from build123d import *

# Parameters (mm, degrees)
SKETCH001_R = 2.2
PAD_DEPTH   = 3
FILLET_R    = 5


with BuildPart() as part:
    # Sketch001 → Pad (new body)
    with BuildSketch(Plane.XY):
        Polygon((3.9, -6), (-3.9, -6), (-3.9, -2), (-5.9, -2), (-5.9, 13), (5.9, 13), (5.9, -2), (3.9, -2), align=None)
        with Locations((0, 8.2)):
            Circle(SKETCH001_R, mode=Mode.SUBTRACT)
        with Locations((0, 2.2)):
            Circle(SKETCH001_R, mode=Mode.SUBTRACT)
    extrude(amount=PAD_DEPTH)

    # Fillet
    fillet_edges = [part.edges().sort_by_distance(p)[0] for p in [
        (5.9, 13, 1.5),
        (-5.9, 13, 1.5),
    ]]
    fillet(fillet_edges, radius=FILLET_R)


solid = part.part
Source: CAD feature listing. Evaluate the final solid. Frame: model axes, mm. A direction names the side the tool comes from. Coordinates: 2 decimals unless noted, no trailing zeros. Order: outer loops, then holes, each group sorted by start corner. A loop starts at its lowest first (then second) coordinate and runs counter-clockwise, first axis right, second up. Notation, with made-up numbers: M 1,73 L 33,73 A9 ccw 33,83 Z; hole C 44,15.5 d10. An arc over 180 degrees is marked long. Write each question's results on one line, items separated by ' | '. Start each with the question number.
1. Section A-A, the plane z = 1.15. Return the cut outline in (x, y), then the cut area to 3 significant figures.
2. Reachability of faces 4 (the face through (-4.47, 11.5, 1.52)), 5 (the face through (3.9, -4, 1)), 6 (the face through (-5, -2, 1)) from +Z, -Z, +X, -X, +Y, -Y: full face, straight path, thin tool, end or side. Return the list, or none.
3. Section C-C, the plane y = 2.2. Return the cut outline in (x, z).
4. Section B-B, the plane x = 0. Return the cut outline in (y, z).
5. Section D-D, the plane y = 6.25. Return the cut outline in (x, z).
6. Draft query along Y for faces 1 (the face through (5, -2, 1)), 2 (the face through (-5.9, 3, 1)), 3 (the face through (0, 6, 1)). Return one class per face: +Y half, -Y half, draft (parallel to the pull), parting line (faces both ways), or undercut.
7. Pin query (flat end, axial travel): pin 1 (0.9 mm diameter, centred on y = -4.5, z = 2, fed in from -X); pin 2 (0.6 mm diameter, centred on x = 4.5, z = 1, fed in from -Y); pin 3 (1.5 mm diameter, centred on y = -3.5, z = 1.5, fed in from +X). Return the tip coordinate at first contact, or that it passes through.
8. Material intervals for L1, parallel to Y at x = 0, z = 1.8; L2, parallel to Y at x = 1, z = 0.8; L3, parallel to X at y = -3.75, z = 2.9, sorted ascending.
Solution:
1) outline: M -5.9,-2 L -3.9,-2 L -3.9,-6 L 3.9,-6 L 3.9,-2 L 5.9,-2 L 5.9,8 A5 ccw 0.9,13 L -0.9,13 A5 ccw -5.9,8 Z; hole C 0,2.2 d4.4; hole C 0,8.2 d4.4 | area: 167 mm²
2) face 4: +Z, -Z, -X, +Y | face 5: +Z, -Z, +X, -Y | face 6: +Z, -Z, -X, -Y
3) outline: M -5.9,0 L -2.2,0 L -2.2,3 L -5.9,3 Z; M 2.2,0 L 5.9,0 L 5.9,3 L 2.2,3 Z
4) outline: M -6,0 L 0,0 L 0,3 L -6,3 Z; M 4.4,0 L 6,0 L 6,3 L 4.4,3 Z; M 10.4,0 L 13,0 L 13,3 L 10.4,3 Z
5) outline: M -5.9,0 L -1.02,0 L -1.02,3 L -5.9,3 Z; M 1.02,0 L 5.9,0 L 5.9,3 L 1.02,3 Z
6) face 1: -Y half | face 2: draft | face 3: undercut
7) pin 1: x = -3.9 | pin 2: y = -2 | pin 3: x = 3.9
8) L1: -6 to 0, 4.4 to 6, 10.4 to 13 | L2: -6 to 0.24, 4.16 to 6.24, 10.16 to 13 | L3: -3.9 to 3.9
